Input: part model. Units: mm. Frame: model coordinates. Face numbers are marked on the shaded views. Round coordinates to 2 decimals unless told otherwise and drop trailing zeros. Write each loop counter-clockwise with the first axis right and the second up, starting at its lowest first coordinate (ties: lowest second). Pieces come first, ordered by that corner, then holes. Notation, with made-up numbers: (-32, -24.75) -> (-5, -24.75) arc R10 ccw to (-5, -9.75) -> close; hole circle Ø8 at (4.25, 37.5). An arc over 180 degrees is marked (long way). Write item = value, one per line.
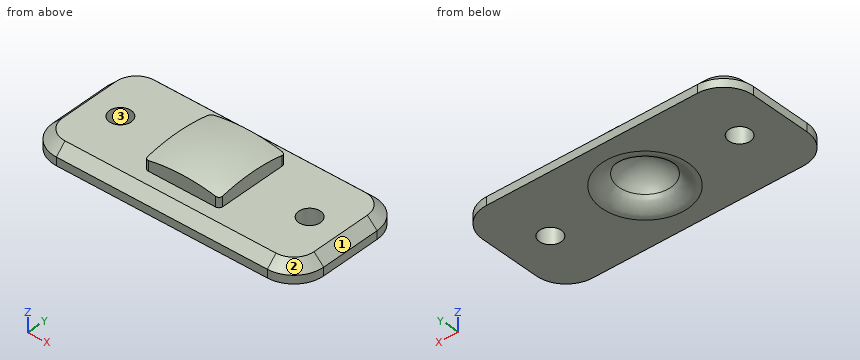
```python
from build123d import *

# Parameters (mm, degrees)
IZIM1_R                     = 1.45
Y_KSEKLIK_EKSTR_ZYON1_DEPTH = 2.4
Y_KSEKLIK_EKSTR_ZYON2_DEPTH = 2.35
PAH1_SIZE                   = 1.3
RADYUS1_R                   = 2.5


with BuildPart() as part:
    # Çizim1 → Yükseklik-Ekstrüzyon1 (new body)
    with BuildSketch(Plane.XY):
        with BuildLine():
            Line((-14.1, 8.045), (14.1, 8.045))
            ThreePointArc((14.1, 8.045), (16.928427125, 6.873427125), (18.1, 4.045))
            Line((18.1, 4.045), (18.1, -4.045))
            ThreePointArc((18.1, -4.045), (16.928427125, -6.873427125), (14.1, -8.045))
            Line((14.1, -8.045), (-14.1, -8.045))
            ThreePointArc((-14.1, -8.045), (-16.928427125, -6.873427125), (-18.1, -4.045))
            Line((-18.1, -4.045), (-18.1, 4.045))
            ThreePointArc((-18.1, 4.045), (-16.928427125, 6.873427125), (-14.1, 8.045))
        make_face()
        with Locations((-12.65, 0)):
            Circle(IZIM1_R, mode=Mode.SUBTRACT)
        with Locations(Location((12.65, 0, 0), (0, 0, 180))):
            Circle(IZIM1_R, mode=Mode.SUBTRACT)
    extrude(amount=Y_KSEKLIK_EKSTR_ZYON1_DEPTH)

    # Çizim2 → Yükseklik-Ekstrüzyon2 (add)
    with BuildSketch(Plane.XY.offset(2.4)):
        with BuildLine():
            Line((-4.5, 5), (4.5, 5))
            ThreePointArc((4.5, 5), (4.853553391, 4.853553391), (5, 4.5))
            Line((5, 4.5), (5, -4.5))
            ThreePointArc((5, -4.5), (4.853553391, -4.853553391), (4.5, -5))
            Line((4.5, -5), (-4.5, -5))
            ThreePointArc((-4.5, -5), (-4.853553391, -4.853553391), (-5, -4.5))
            Line((-5, -4.5), (-5, 4.5))
            ThreePointArc((-5, 4.5), (-4.853553391, 4.853553391), (-4.5, 5))
        make_face()
    extrude(amount=Y_KSEKLIK_EKSTR_ZYON2_DEPTH)

    # Çizim3 → Kes-Döndür1 (revolve, cut)
    with BuildSketch(Plane(origin=(0, 0, 0), x_dir=(1, 0, 0), z_dir=(0, 1, 0))):
        with BuildLine():
            Line((0, -8.133060599), (11.181129459, -8.714892386))
            Line((11.181129459, -8.714892386), (7.979795791, -3.321493976))
            ThreePointArc((7.979795791, -3.321493976), (4.05332488, -4.390057277), (0, -4.75))
            Line((0, -4.75), (0, -8.133060599))
        make_face()
        with BuildLine():
            Line((3.765, 0), (5.976478481, 3.08469305))
            Line((5.976478481, 3.08469305), (3.765, 3.765))
            Line((3.765, 3.765), (0, 3.765))
            Line((0, 3.765), (0, -3.765))
            ThreePointArc((0, -3.765), (2.662257031, -2.662257031), (3.765, 0))
        make_face()
    revolve(axis=Axis((0, 0, 8.133060599), (0, 0, -1)), mode=Mode.SUBTRACT)

    # Pah1
    pah1_edges = [part.edges().sort_by_distance(p)[0] for p in [
        (16.928427125, -6.873427125, 2.4),
        (18.1, 0, 2.4),
        (16.928427125, 6.873427125, 2.4),
        (0, 8.045, 2.4),
        (-16.928427125, 6.873427125, 2.4),
        (-18.1, 0, 2.4),
        (-16.928427125, -6.873427125, 2.4),
        (0, -8.045, 2.4),
    ]]
    chamfer(pah1_edges, length=PAH1_SIZE)

    # Radyus1
    radyus1_edges = [part.edges().sort_by_distance(p)[0] for p in [
        (-3.765, 0, 0),
    ]]
    fillet(radyus1_edges, radius=RADYUS1_R)


solid = part.part
```
1) Line query: L1, parallel to Y at x = 12.65, z = 0.75 (3 decimals); L2, parallel to Z at x = 6, y = 0; L3, parallel to X at y = 2.5, z = 1.3. Output: solid intervals per line, ascending. Write a range as from..to.
Solutions:
L1 = -8.045..-1.45, 1.45..8.045
L2 = 0..2.4
L3 = -17.9..-2.52, 2.52..17.9
2) Cut plane D-D (x = -7.5). Return the cut outline in (y, z) (3 decimals).
Solutions:
outline = (-8.045, 0) -> (8.045, 0) -> (8.045, 1.1) -> (6.745, 2.4) -> (-6.745, 2.4) -> (-8.045, 1.1) -> close
3) Draft query along Y for the marked faces 1, 2 and 3. Return one class per face: +Y half, -Y half, draft (parallel to the pull), parting line (faces both ways), or undercut.
Solutions:
face_1 = draft
face_2 = -Y half
face_3 = undercut
4) Cut plane C-C (y = 0). Count the separate pieces of the cut face and the enclosed holes in it, and give its area (3 significant figures).
Solutions:
separate_pieces = 3
enclosed_holes = 0
area = 69.4 mm^2
5) Cut plane B-B (z = 1.95). Return the cut outline in (x, y) (3 decimals).
Solutions:
outline = (-17.25, -4.045) arc R3.15 ccw to (-14.1, -7.195) -> (14.1, -7.195) arc R3.15 ccw to (17.25, -4.045) -> (17.25, 4.045) arc R3.15 ccw to (14.1, 7.195) -> (-14.1, 7.195) arc R3.15 ccw to (-17.25, 4.045) -> close; hole circle Ø2.9 at (-12.65, 0); hole circle Ø6.441 at (0, 0); hole circle Ø2.9 at (12.65, 0)
6) First-contact query: P1, Ø4, axis at x = 5, y = 3.5, coming from the +Z side; P2, Ø1.5, axis at y = -6, z = 1.5, coming from the +X side; P3, Ø4, axis at x = 13, y = 3.5, coming from the +Z side; P4, Ø2.5, axis at x = -12.65, y = 0, coming from the +Z side. Flat tips, straight axial feed; report the tip coordinate or a pass-through.
Solutions:
P1 = 4.38
P2 = 17.88
P3 = 2.4
P4 = through
7) Cut plane A-A (x = -12.65). Return the cut outline in (y, z) (3 decimals), and give its area (3 significant figures).
Solutions:
outline = (-8.045, 0) -> (-1.45, 0) -> (-1.45, 2.4) -> (-6.745, 2.4) -> (-8.045, 1.1) -> close; (1.45, 0) -> (8.045, 0) -> (8.045, 1.1) -> (6.745, 2.4) -> (1.45, 2.4) -> close
area = 30.0 mm^2
